from build123d import *

# Parameters (mm, degrees)
SKETCH1_W           = 116
SKETCH1_H           = 96
BOSS_EXTRUDE1_DEPTH = 2
SKETCH2_W           = 2
SKETCH2_H           = 4
BOSS_EXTRUDE2_DEPTH = 5.5
SKETCH3_W           = 2
SKETCH3_H           = 2
BOSS_EXTRUDE3_DEPTH = 2
CHAMFER2_SIZE       = 5


with BuildPart() as part:
    # Sketch1 → Boss-Extrude1 (new body)
    with BuildSketch(Plane(origin=(0, 0, 0), x_dir=(1, 0, 0), z_dir=(0, 1, 0))):
        Rectangle(SKETCH1_W, SKETCH1_H)
    extrude(amount=BOSS_EXTRUDE1_DEPTH)

    # Sketch2 → Boss-Extrude2 (add)
    with BuildSketch(Plane(origin=(0, 2, 0), x_dir=(1, 0, 0), z_dir=(0, 1, 0))):
        with Locations((54, -36.5)):
            Rectangle(SKETCH2_W, SKETCH2_H)
        with Locations((54, 33.5)):
            Rectangle(SKETCH2_W, SKETCH2_H)
    boss_extrude2 = extrude(amount=BOSS_EXTRUDE2_DEPTH)

    # Sketch3 → Boss-Extrude3 (add)
    with BuildSketch(Plane(origin=(55, 0, 0), x_dir=(0, 0, -1), z_dir=(1, 0, 0))):
        with Locations((-36.5, 6.5)):
            Rectangle(SKETCH3_W, SKETCH3_H)
        with Locations((33.5, 6.5)):
            Rectangle(SKETCH3_W, SKETCH3_H)
    boss_extrude3 = extrude(amount=BOSS_EXTRUDE3_DEPTH)

    # Mirror1: Boss-Extrude2, Boss-Extrude3 across plane
    add(boss_extrude2.mirror(Plane(origin=(0, 0, 0), x_dir=(0, 0, 1), z_dir=(1, 0, 0))))
    add(boss_extrude3.mirror(Plane(origin=(0, 0, 0), x_dir=(0, 0, 1), z_dir=(1, 0, 0))))

    # Chamfer2
    chamfer2_edges = [part.edges().sort_by_distance(p)[0] for p in [
        (53, 2, 36.5),
        (53, 2, -33.5),
        (-53, 2, 36.5),
        (-53, 2, -33.5),
    ]]
    chamfer(chamfer2_edges, length=CHAMFER2_SIZE)


solid = part.part
The listing builds one solid part. Answer for the finished solid, in the listing's coordinates (mm). A direction names the side the tool comes from. Give positions to 0.01 mm unless a question says otherwise; leave off trailing zeros. Loops run counter-clockwise (first coordinate to the right, second up) from the corner with the lowest first, then second, coordinate; pieces in that order, holes last. Notation, with made-up numbers: M 84,86.25 L 126,86.25 A9 cw 126,96.25 Z; hole C -23.5,44 d6. An arc over 180 degrees is marked long. Answer as CSV lines item,"result".
Item 1: The mould has two halves that part along X. Classify faces 1 (the flat face through (-51, 5, 37)), 2 (the flat face through (-52, 4, 38.5)): released by +X, released by -X, zero draft, split by the parting line, or undercut.
Values follow:
face 1,"undercut"
face 2,"zero draft"
Item 2: Given pin 1 Ø1.6 at (x, y) = (56.5, 6.5) entering from -Z; pin 2 Ø0.6 at (y, z) = (6.5, -33.5) entering from +X; pin 3 Ø1.6 at (x, y) = (-52.5, 4) entering from +Z, each flat-ended and moving along its own axis, determine where each tip first touches the part or whether it passes through.
Values follow:
pin 1,"stops at z = -34.5"
pin 2,"stops at x = 57"
pin 3,"stops at z = 38.5"
Item 3: Which of the six approach directions +Z, -Z, +X, -X, +Y, -Y give full straight-line access (tool end or side, diameter ignored) to faces 3 (the flat face through (-52, 4, -35.5)), 4 (the flat face through (51, 5, 37)), 5 (the flat face through (52, 4, -31.5))?
Values follow:
face 3,"-Z, +X, -X, +Y"
face 4,"+Z, -Z, +Y"
face 5,"+X, -X, +Y"
Item 4: The part is cut by section B-B (z = -23). Give the vertices of the cut face in (x, y).
Values follow:
outline,"M -58,0 L 58,0 L 58,2 L -58,2 Z"
Item 5: The part is cut by section A-A (x = -18). Give the vertices of the cut face in (y, z).
Values follow:
outline,"M 0,-48 L 2,-48 L 2,48 L 0,48 Z"
Item 6: Straight lines are drawn through the part: line 1 along Y through (x, z) = (-23, -27.5); line 2 along X through (y, z) = (3.5, -32). For each, find the intervals that lie inside material, in ascending order. Write a range as [from, to].
Values follow:
line 1,"y = [0, 2]"
line 2,"x = [-55, -49.5], [49.5, 55]"
